The model under review builds one solid part; all positions refer to its coordinate system, in mm. A direction names the side the tool comes from. Coordinates: 2 decimals unless noted, no trailing zeros. Loops run counter-clockwise (first coordinate to the right, second up) from the corner with the lowest first, then second, coordinate; pieces in that order, holes last. Notation, with made-up numbers: (-11.5, 25) - (18.5, 25) arc R27 cw to (18.5, 62) - close; hole circle Ø5 at (64, 33.5). An arc over 180 degrees is marked (long way). Use a Markdown table: item, result. Add a question column.
1) For faces 5 (the flat face through (13, 51, 5)), 6 (the flat face through (15, 34.5, -2.6)), 7 (the flat face through (23, 27, 0)), 8 (the flat face through (19, 15, 0)), list the 3-axis set-ups (+Z, -Z, +X, -X, +Y, -Y) from which the entire face can be reached by the end or side of a thin tool; tool diameter is ignored.
2) Clearance check with flat-ended pins moving along their axes: pin 1 (1.5 mm diameter, centred on x = -13.5, z = -10, fed in from +Y); pin 2 (24.5 mm diameter, centred on y = 87, z = 0, fed in from -X); pin 3 (12 mm diameter, centred on x = 28, z = -18, fed in from +Y). State where each tip first meets the part, or that it passes through.
3) Add section C-C, the plane z = -24.5. Give the boundary of the cut face in (x, y), and give its area (3 significant figures).
4) The part is to be moulded in two halves that separate along Z. For faces 1 (the cylindrical face through (-17.028, 33.993, 0.66)), 2 (the cylindrical face through (16.972, 33.993, 0.66)), 3 (the flat face through (2.5, 63, 11)), 4 (the flat face through (-0.107, 46.234, -22.314)), say which applies: pulls with the +Z half, pulls with the -Z half, needs draft (parallel to the pull), parting line crosses it, or undercut.
5) To check wall thickness, follow L1, parallel to Z at x = 26, y = 87; L2, parallel to X at y = 22, z = 7.5; L3, parallel to X at y = 35.5, z = 3.5. State the ranges of each line that lie inside material, in increasing order. Write a range as [from, to].
6) Add section D-D, the plane x = -0.5. Give the boundary of the cut face in (y, z).
7) Add section A-A, the plane x = 17.5. Give the boundary of the cut face in (y, z), and give its area (3 significant figures).
8) Add section B-B, the plane y = 87. Give the boundary of the cut face in (x, z).
Autodesk Inventor part; units mm, degrees
ref_plane "YZ Plane" through (0, 0, 0) normal (1, 0, 0) x (0, 1, 0)
ref_plane "XZ Plane" through (0, 0, 0) normal (0, 1, 0) x (-1, 0, 0)
ref_plane "XY Plane" through (0, 0, 0) normal (0, 0, 1) x (1, 0, 0)
sketch "Sketch1" plane through (0, 0, 0) normal (1, 0, 0) x (0, 1, 0)
  line L0 (0, 33) -> (0, -33)
  line L1 (47.2724, 0) -> (-31.6075, 0)
  line L2 (0, 33) -> (4, 33)
  line L3 (4, 33) -> (4, -33)
  line L4 (4, -33) -> (0, -33)
  line L5 (87, 12) -> (87, -12)
  line L6 (87, 12) -> (4, 33)
  line L7 (87, -12) -> (4, -33)
  line L8 (51, 21.1084) -> (51, -21.1084)
  circle A0 centre (4, 0) radius 24 construction
  circle A1 centre (4, 0) radius 30 construction
  arc A2 (4, -24) -> (4, 24) centre (4, 0) ccw
  arc A3 (4, -30) -> (4, 30) centre (4, 0) ccw
  point P0 (0, 0)
  dimension "d9" = 48
  dimension "d0" = 66
  dimension "d1" = 4
  dimension "d2" = 24
  dimension "d3" = 87
  dimension "d4" = 36
  dimension "d10" = 60
extrude "Extrusion1" add sketch "Sketch1" along normal mid plane 46 contours L6 L8 L7 L3 A3 | L3 A2 L1 | L1 A2 L3 | A3 L1 A2 L3 | L1 A3 L3 A2
extrude "Extrusion2" add sketch "Sketch1" along normal mid plane 5 contours L6 L5 L7 L8
sketch "Sketch2" plane through (0, 0, 0) normal (0, 0, 1) x (1, 0, 0)
  line L0 (-2.5, 87) -> (2.5, 87)
  line L1 (0, 87) -> (0, 0)
  line L2 (-15, 44) -> (15, 44)
  line L3 (15, 44) -> (15, 4)
  line L4 (15, 4) -> (-15, 4)
  line L5 (-15, 4) -> (-15, 44)
  line L6 (-23, 4) -> (23, 4)
  dimension "d13" = 30
  dimension "d14" = 40
extrude "Extrusion4" cut sketch "Sketch2" along normal mid plane 66
sketch "Sketch3" plane through (0, 0, 0) normal (1, 0, 0) x (0, 1, 0)
  line L0 (87, -12) -> (87, 12)
  circle A0 centre (87, 0) radius 9.5
  circle A1 centre (87, 0) radius 14
  point P0 (0, 0)
  dimension "d17" = 19
  dimension "d18" = 28
extrude "Extrusion5" add sketch "Sketch3" along normal blind 51 and the other way blind 5
sketch "Sketch4" plane through (0, 0, 0) normal (1, 0, 0) x (0, 1, 0)
  line L0 (87, 9.5) -> (87, -9.5)
  circle A0 centre (87, 0) radius 9.5
  point P0 (0, 0)
extrude "Extrusion6" cut sketch "Sketch4" along normal blind 51 and the other way blind 5 contours L0 A0 picked at (82.8782, 1.7989)
extrude "Extrusion7" cut sketch "Sketch1" along normal mid plane 38 contours L3 A2 L1 | L1 A2 L3 | A3 L1 A2 L3 | L1 A3 L3 A2
sketch "Sketch5" plane through (0, 0, 0) normal (0, 0, 1) x (1, 0, 0)
  line L0 (2.5, 73) -> (19.5, 73)
  line L1 (19.5, 73) -> (19.5, 51)
  line L2 (19.5, 51) -> (2.5, 51)
  line L3 (2.5, 51) -> (2.5, 73)
  line L4 (23, 51) -> (2.5, 51) construction
  line L5 (2.5, 51) -> (0, 51) construction
  line L6 (0, 87.0731) -> (77.1013, 87.0731) construction
  line L7 (0, 87.0731) -> (36, 87.0731)
  point P0 (0, 0)
  dimension "d29" = 22
  dimension "d30" = 17
  dimension "d31" = 36
extrude "Extrusion8" add sketch "Sketch5" along normal mid plane 3
sketch "Sketch6" plane through (19.5, 51, 1.5) normal (1, 0, 0) x (0, 0, -1)
  point P0 (1.5, -51)
sketch "Sketch7" plane through (-5, 87, 0) normal (-1, 0, 0) x (0, 0, 1)
  point P0 (0, -87)
sketch "Sketch8" plane through (0, 0, 0) normal (0, 0, 1) x (1, 0, 0)
  line L0 (-5, 101) -> (-5, 73) construction
  line L1 (-5, 87) -> (51, 87)
  line L2 (51, 73) -> (51, 101) construction
  point P0 (0, 0)
sketch "Sketch9" plane through (23, 0, 0) normal (1, 0, 0) x (0, 0, -1)
  point P0 (0, 0)
sketch "Sketch10" plane through (51, 87, 0) normal (1, 0, 0) x (0, 0, -1)
  circle A0 centre (0, 0) radius 14
  line L0 (-14, 0) -> (14, 0) construction
  point P0 (0, -87)
sketch "Sketch11" plane through (-5, 87, 0) normal (-1, 0, 0) x (0, 0, 1)
  circle A0 centre (0, 0) radius 14
  line L0 (-14, 0) -> (14, 0) construction
  point P0 (0, -87)
properties part number "Bai_16"
From the geometry:
| question | item | result |
|---|---|---|
| 1 | face 5 | +X |
| 1 | face 6 | +Z, -Z, -Y |
| 1 | face 7 | +Z, -Z, +X, -Y |
| 1 | face 8 | -Y |
| 2 | pin 1 | stops at y = 51 |
| 2 | pin 2 | stops at x = -5 |
| 2 | pin 3 | stops at y = 94.21 |
| 3 | outline | (-23, 4) - (-19, 4) - (-19, 21.31) - (-15, 21.31) - (-15, 37.6) - (-23, 37.6) - close; (15, 21.31) - (19, 21.31) - (19, 4) - (23, 4) - (23, 37.6) - (15, 37.6) - close |
| 3 | area | 399 mm^2 |
| 4 | face 1 | undercut |
| 4 | face 2 | undercut |
| 4 | face 3 | needs draft |
| 4 | face 4 | pulls with the -Z half |
| 5 | L1 | z = [-14, -9.5], [9.5, 14] |
| 5 | L2 | x = [-23, -19], [19, 23] |
| 5 | L3 | x = [-23, -15], [15, 23] |
| 6 | outline | (44, -22.88) - (82.3, -13.19) arc R14 ccw (long way) to (82.3, 13.19) - (44, 22.88) - close; hole circle Ø19 at (87, 0) |
| 7 | outline | (4, -33) - (51, -21.11) - (51, -1.5) - (73, -1.5) - (73, 1.5) - (51, 1.5) - (51, 21.11) - (4, 33) - (4, 30) arc R30 cw to (4, -30) - close; circle Ø28 at (87, 0); hole circle Ø19 at (87, 0) |
| 7 | area | 1,530 mm^2 |
| 8 | outline | (-5, -14) - (51, -14) - (51, -9.5) - (-5, -9.5) - close; (-5, 9.5) - (51, 9.5) - (51, 14) - (-5, 14) - close |
